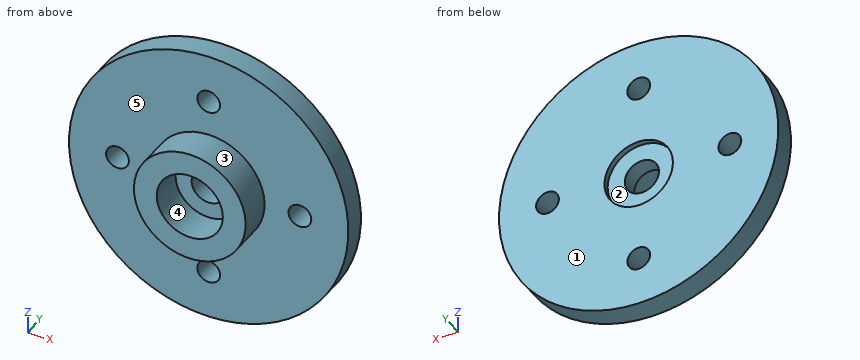
from build123d import *

# Parameters (mm, degrees)
SKETCH_1_R          = 12.25
SKETCH_1_R_2        = 3
SKETCH_1_R_3        = 1
SKETCH_1_R_4        = 2.9
SKETCH_1_R_5        = 1.5
EXTRUDE_1_DEPTH     = 2
SKETCH_2_R          = 4.9
SKETCH_2_R_2        = 2.9
EXTRUDE_2_DEPTH     = 3
CUT_EXTRUDE_START   = 2
SKETCH_1_4_R        = 3
CUT_EXTRUDE_1_DEPTH = 0.5


with BuildPart() as part:
    # 草图1 → 凸台-拉伸1 (new body)
    # profile 1 of 3: a face of its own
    with BuildSketch(Plane(origin=(0, 0, 0), x_dir=(1, 0, 0), z_dir=(0, 1, 0))):
        with Locations(Location((0, 0, 0), (0, 0, 270))):
            Circle(SKETCH_1_R)
        Circle(SKETCH_1_R_2, mode=Mode.SUBTRACT)
        with Locations(Location((-8, 0, 0), (0, 0, 270))):
            Circle(SKETCH_1_R_3, mode=Mode.SUBTRACT)
        with Locations(Location((0, -8, 0), (0, 0, 270))):
            Circle(SKETCH_1_R_3, mode=Mode.SUBTRACT)
        with Locations(Location((8, 0, 0), (0, 0, 270))):
            Circle(SKETCH_1_R_3, mode=Mode.SUBTRACT)
        with Locations(Location((0, 8, 0), (0, 0, 270))):
            Circle(SKETCH_1_R_3, mode=Mode.SUBTRACT)
    # profile 2 of 3: a face of its own
    with BuildSketch(Plane(origin=(0, 0, 0), x_dir=(1, 0, 0), z_dir=(0, 1, 0))):
        Circle(SKETCH_1_R_2)
        Circle(SKETCH_1_R_4, mode=Mode.SUBTRACT)
    # profile 3 of 3: a face of its own
    with BuildSketch(Plane(origin=(0, 0, 0), x_dir=(1, 0, 0), z_dir=(0, 1, 0))):
        Circle(SKETCH_1_R_4)
        with Locations(Location((0, 0, 0), (0, 0, 270))):
            Circle(SKETCH_1_R_5, mode=Mode.SUBTRACT)
    extrude(amount=EXTRUDE_1_DEPTH)

    # 草图2 → 凸台-拉伸2 (add)
    with BuildSketch(Plane.XZ):
        with Locations(Location((0, 0, 0), (0, 0, 90))):
            Circle(SKETCH_2_R)
        with Locations(Location((0, 0, 0), (0, 0, 270))):
            Circle(SKETCH_2_R_2, mode=Mode.SUBTRACT)
    extrude(amount=EXTRUDE_2_DEPTH)

    # 草图1<4> → 切除-拉伸1 (cut)
    with BuildSketch(Plane(origin=(0, 0, 0), x_dir=(1, 0, 0), z_dir=(0, 1, 0)).offset(CUT_EXTRUDE_START)):
        with Locations(Location((0, 0, 0), (0, 0, 270))):
            Circle(SKETCH_1_4_R)
    extrude(amount=-CUT_EXTRUDE_1_DEPTH, mode=Mode.SUBTRACT)


solid = part.part
Geometry: final body of the model. Coordinates: model frame, mm. Face numbers are marked on the shaded views. A direction names the side the tool comes from. Give positions to 0.01 mm unless a question says otherwise; leave off trailing zeros. Write each loop counter-clockwise with the first axis right and the second up, starting at its lowest first coordinate (ties: lowest second). Pieces come first, ordered by that corner, then holes.
(1) Ray query, line 1 (X direction, y = 0.45, z = 0); line 2 (Y direction, x = -5, z = -11); line 3 (Z direction, x = -0.75, y = 1.2). Return the intervals inside material, ascending.
(2) First-contact query: P1, Ø3, axis at x = -1.5, z = 0.5, coming from the -Y side; P2, Ø5, axis at x = 0, z = 0, coming from the -Y side; P3, Ø1, axis at x = -3, y = -2, coming from the -Z side. Flat tips, straight axial feed; report the tip coordinate or a pass-through.
(3) Access query for the marked faces 1 and 2. Directions: +Z, -Z, +X, -X, +Y, -Y. A direction counts if a zero-diameter tool reaches every point of the face in a straight line with its end or side. Return the directions, or none.
(4) Mould query, pull axis X, two halves, no side actions, for the marked faces 3, 4 and 5. Classes: released by +X, released by -X, zero draft, split by the parting line, or undercut.
(5) Cut plane B-B, the plane y = 0.7. Return loops of the section in (x, z), then the cut area to 3 significant figures.
(6) Cut plane C-C, the plane z = 8. Return loops of the section in (x, y).
(7) Cut plane D-D, the plane x = -3.75. Return loops of the section in (y, z).
(8) Cut plane A-A, the plane x = -8. Return loops of the section in (y, z), then the cut area to 3 significant figures.
Values follow:
1. line 1: x = -12.25 to -9, -7 to -1.5, 1.5 to 7, 9 to 12.25
1. line 2: y = 0 to 2
1. line 3: z = -12.23 to -8.66, -7.34 to -1.3, 1.3 to 7.34, 8.66 to 12.23
2. P1: stops at y = -3
2. P2: stops at y = 0
2. P3: stops at z = -4.21
3. face 1: +Z, -Z, +X, -X, +Y
3. face 2: +Y
4. face 3: split by the parting line
4. face 4: undercut
4. face 5: zero draft
5. outline: circle Ø24.5 at (0, 0); hole circle Ø2 at (-8, 0); hole circle Ø3 at (0, 0); hole circle Ø2 at (0, -8); hole circle Ø2 at (0, 8); hole circle Ø2 at (8, 0)
5. area: 452 mm2
6. outline: (-9.28, 0) - (-1, 0) - (-1, 2) - (-9.28, 2) - close; (1, 0) - (9.28, 0) - (9.28, 2) - (1, 2) - close
7. outline: (-3, -3.15) - (0, -3.15) - (0, -11.66) - (2, -11.66) - (2, 11.66) - (0, 11.66) - (0, 3.15) - (-3, 3.15) - close
8. outline: (0, -9.28) - (2, -9.28) - (2, -1) - (0, -1) - close; (0, 1) - (2, 1) - (2, 9.28) - (0, 9.28) - close
8. area: 33.1 mm2
